```python
from build123d import *

# Parameters (mm, degrees)
F0_R     = 4
F1_DEPTH = 2.4
F2_D     = 3.6
F3_R     = 0.2


with BuildPart() as f1:
    # F0 (on Top) → F1 (new body)
    with BuildSketch(Plane.XY):
        Circle(F0_R)
    extrude(amount=F1_DEPTH)

    # F2 (through all)
    with Locations(Plane(origin=(0, 0, 0), x_dir=(1, 0, 0), z_dir=(0, 0, -1))):
        with Locations((0, 0)):
            Hole(F2_D / 2)

    # F3
    f3_edges = [f1.edges().sort_by_distance(p)[0] for p in [
        (-4, 0, 2.4),
        (-1.8, 0, 2.4),
    ]]
    fillet(f3_edges, radius=F3_R)


solid = f1.part
```
Read the model definition and answer for the solid it produces. Units are mm, in the model's axes. Round coordinates to 2 decimals unless told otherwise and drop trailing zeros. Write each loop counter-clockwise with the first axis right and the second up, starting at its lowest first coordinate (ties: lowest second). Pieces come first, ordered by that corner, then holes. Notation, with made-up numbers: M 44.5,-10 L 53.5,-10 A28 ccw 53.5,12 Z; hole C -21,0.5 d3. An arc over 180 degrees is marked long. One line per item, written item: value.
Q1. Straight lines are drawn through the part: line 1 (Y direction, x = 0, z = 1.7); line 2 (X direction, y = 1.5, z = 1.8); line 3 (X direction, y = 0.5, z = 0.45). For each, find the intervals that lie inside material, in ascending order. Write a range as [from, to].
Data:
line 1: [-4, -1.8], [1.8, 4]
line 2: [-3.71, -0.99], [0.99, 3.71]
line 3: [-3.97, -1.73], [1.73, 3.97]
Q2. Find section C-C on z = 0.8. Write down the section's boundary in (x, y).
Data:
outline: C 0,0 d8; hole C 0,0 d3.6
Q3. Find section A-A on x = 0. Write down the section's boundary in (y, z).
Data:
outline: M -4,0 L -1.8,0 L -1.8,2.2 A0.2 ccw -2,2.4 L -3.8,2.4 A0.2 ccw -4,2.2 Z; M 1.8,0 L 4,0 L 4,2.2 A0.2 ccw 3.8,2.4 L 2,2.4 A0.2 ccw 1.8,2.2 Z
Q4. For a pull along Y with two mould halves and no side action, classify faces 1 (the flat face through (2, -1, 0)), 2 (the cylindrical face through (-1.717, -0.541, 1.115)), 3 (the cylindrical face through (-0.867, -3.905, 1.085)) as +Y half, -Y half, draft (parallel to the pull), parting line (faces both ways), or undercut.
Data:
face 1: draft
face 2: undercut
face 3: parting line
